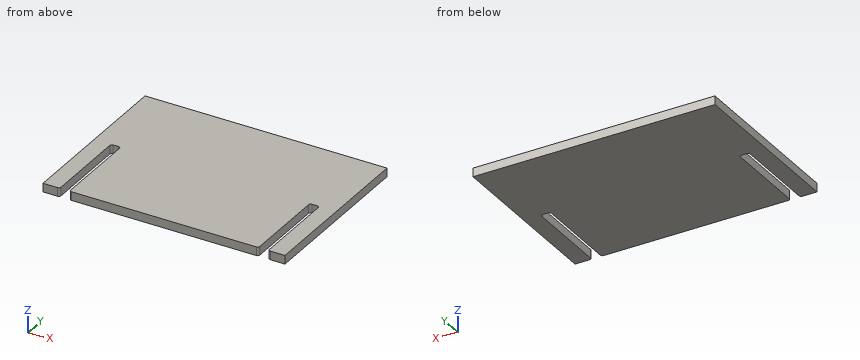
```python
from build123d import *

# Parameters (mm, degrees)
BOSS_EXTRUDE1_DEPTH = 6.35
MOVE_FACE_SLOT_BY   = 0.762
MOVE_FACE_SLOT_2_BY = 0.762
MOVE_FACE_SLOT_3_BY = 0.762
MOVE_FACE_SLOT_4_BY = 0.762
MOVE_FACE_SLOT_5_BY = 0.762
MOVE_FACE_SLOT_6_BY = 0.762
FILLET1_R           = 3.175


with BuildPart() as part:
    # Sketch1 → Boss-Extrude1 (new, symmetric)
    with BuildSketch(Plane.XY):
        Polygon((1294.203955658, -24.179867224), (1649.803955658, -24.179867224), (1649.803955658, -278.179867224), (1624.403955658, -278.179867224), (1624.403955658, -151.179867224), (1611.703955658, -151.179867224), (1611.703955658, -278.179867224), (1332.303955658, -278.179867224), (1332.303955658, -151.179867224), (1319.603955658, -151.179867224), (1319.603955658, -278.179867224), (1294.203955658, -278.179867224), align=None)
    extrude(amount=BOSS_EXTRUDE1_DEPTH, both=True)

    # Move Face slot: a face moved inward by 0.762
    extrude(part.faces().sort_by_distance((1611.703955658, -214.679867224, 0))[0], amount=MOVE_FACE_SLOT_BY, dir=(-1, 0, 0), mode=Mode.SUBTRACT)

    # Move Face slot 2: a face moved inward by 0.762
    extrude(part.faces().sort_by_distance((1624.403955658, -214.679867224, 0))[0], amount=MOVE_FACE_SLOT_2_BY, dir=(1, 0, 0), mode=Mode.SUBTRACT)

    # Move Face slot 3: a face moved inward by 0.762
    extrude(part.faces().sort_by_distance((1618.053955658, -151.179867224, 0))[0], amount=MOVE_FACE_SLOT_3_BY, dir=(0, 1, 0), mode=Mode.SUBTRACT)

    # Move Face slot 4: a face moved inward by 0.762
    extrude(part.faces().sort_by_distance((1332.303955658, -214.679867224, 0))[0], amount=MOVE_FACE_SLOT_4_BY, dir=(1, 0, 0), mode=Mode.SUBTRACT)

    # Move Face slot 5: a face moved inward by 0.762
    extrude(part.faces().sort_by_distance((1325.953955658, -151.179867224, 0))[0], amount=MOVE_FACE_SLOT_5_BY, dir=(0, 1, 0), mode=Mode.SUBTRACT)

    # Move Face slot 6: a face moved inward by 0.762
    extrude(part.faces().sort_by_distance((1319.603955658, -214.679867224, 0))[0], amount=MOVE_FACE_SLOT_6_BY, dir=(-1, 0, 0), mode=Mode.SUBTRACT)

    # Fillet1
    fillet1_edges = [part.edges().sort_by_distance(p)[0] for p in [
        (1625.165955658, -278.179867224, 0),
        (1625.165955658, -150.417867224, 0),
        (1610.941955658, -150.417867224, 0),
        (1610.941955658, -278.179867224, 0),
        (1333.065955658, -278.179867224, 0),
        (1333.065955658, -150.417867224, 0),
        (1318.841955658, -150.417867224, 0),
        (1318.841955658, -278.179867224, 0),
    ]]
    fillet(fillet1_edges, radius=FILLET1_R)


solid = part.part
```
CAD build for the part. Positions are in the model's coordinates, mm. Round coordinates to 2 decimals unless told otherwise and drop trailing zeros. Loops run counter-clockwise (first coordinate to the right, second up) from the corner with the lowest first, then second, coordinate; pieces in that order, holes last. Notation, with made-up numbers: (-36.5, -9) - (-25.5, -9) arc R23 cw to (-25.5, 29) - close; hole circle Ø2 at (-36.75, 84.5). An arc over 180 degrees is marked (long way). Return JSON: item names as keys, results as strings. Group by question number.
Q1. Drill centre lines: line 1 along X through (y, z) = (-156, 3.5); line 2 along Y through (x, z) = (1331, -2.5). Where is each one in solid material? Low to high. Write a range as [from, to].
Q2. Band-saw the part on B-B on z = -1. Give the cut face in (x, y) (3 decimals), plus the area to 3 significant figures.
Q3. Band-saw the part on A-A on y = -212.5. Give the cut face in (x, z).
Solutions:
{
 "1": {"line 1": "x = [1294.2, 1318.84], [1333.07, 1610.94], [1625.17, 1649.8]", "line 2": "y = [-150.62, -24.18]"},
 "2": {"outline": "(1294.204, -278.18) - (1315.667, -278.18) arc R3.175 ccw to (1318.842, -275.005) - (1318.842, -153.593) arc R3.175 cw to (1322.017, -150.418) - (1329.891, -150.418) arc R3.175 cw to (1333.066, -153.593) - (1333.066, -275.005) arc R3.175 ccw to (1336.241, -278.18) - (1607.767, -278.18) arc R3.175 ccw to (1610.942, -275.005) - (1610.942, -153.593) arc R3.175 cw to (1614.117, -150.418) - (1621.991, -150.418) arc R3.175 cw to (1625.166, -153.593) - (1625.166, -275.005) arc R3.175 ccw to (1628.341, -278.18) - (1649.804, -278.18) - (1649.804, -24.18) - (1294.204, -24.18) - close", "area": "86,700 mm^2"},
 "3": {"outline": "(1294.2, -6.35) - (1318.84, -6.35) - (1318.84, 6.35) - (1294.2, 6.35) - close; (1333.07, -6.35) - (1610.94, -6.35) - (1610.94, 6.35) - (1333.07, 6.35) - close; (1625.17, -6.35) - (1649.8, -6.35) - (1649.8, 6.35) - (1625.17, 6.35) - close"}
}
